Work out the finished part from the listing and answer in its coordinate system (mm). A direction names the side the tool comes from. Coordinates: 2 decimals unless noted, no trailing zeros. Order: outer loops, then holes, each group sorted by start corner. A loop starts at its lowest first (then second) coordinate and runs counter-clockwise, first axis right, second up. Notation, with made-up numbers: M 88,19.25 L 134,19.25 A23 ccw 134,32.25 Z; hole C 82,-23.75 d2. An arc over 180 degrees is marked long. Write item = value, one per line. Start each with the question number.
Q1. Determine the mould class of faces 6 (the cylindrical face through (-8.218, 0.731, 4.825)), 7 (the flat face through (4.02, -0.01, 6.96)), 8 (the flat face through (-4.02, -0.01, 6.96)), 9 (the flat face through (8, 0, 0)) for opening direction X: released by +X, released by -X, zero draft, split by the parting line, or undercut.
Q2. Find section B-B on y = -0.75. Give the vertices of the cut face in (x, z) (3 decimals).
Q3. A tool of negligible diameter and unlimited length cuts with its end or side. For faces 1 (the flat face through (4.02, -0.01, -6.96)), 2 (the cylindrical face through (0, 0, 6.5)), 3 (the flat face through (-0.1, 1, -4.5)), 4 (the flat face through (-8, 0, 0)), 5 (the flat face through (-4.02, -0.01, -6.96)), from which of +Z, -Z, +X, -X, +Y, -Y can it reach the whole face along a straight path? Write none if from no direction.
Q4. Straight lines are drawn through the part: line 1 along Z through (x, y) = (0, 0.3); line 2 along X through (y, z) = (-0.35, -2.5); line 3 along X through (y, z) = (-0.25, -2). For each, find the intervals that lie inside material, in ascending order.
Q5. Find section A-A on x = 0. Give the vertices of the cut face in (y, z), and give its area (3 significant figures).
Q6. Find section D-D on x = 3.5. Give the number of separate pieces and of enclosed holes in the cut face, and give its area (3 significant figures).
Q7. Each of these flat-tipped pins is pushed along its axis until it touches: P1, Ø9, axis at x = 0, z = 0, coming from the -Y side; P2, Ø1, axis at x = -8, y = -0.5, coming from the -Z side. Where does it stop, or does it pass through?
Q8. Find section C-C on z = -3.5. Give the vertices of the cut face in (x, y).
```python
from build123d import *

# Parameters (mm, degrees)
SKETCH005_R          = 9.53
SKETCH005_R_2        = 4
PAD001_DEPTH         = 1
POCKET001_DEPTH      = 55.059013
POCKET001_DEPTH_BACK = 55.059013
POLARPATTERN_COUNT   = 3
SKETCH007_R          = 0.5


with BuildPart() as part:
    # Sketch005 → Pad001 (new body, symmetric)
    with BuildSketch(Plane.XZ):
        Circle(SKETCH005_R)
        Circle(SKETCH005_R_2, mode=Mode.SUBTRACT)
    extrude(amount=PAD001_DEPTH, both=True)

    # Sketch006 → Pocket001 (cut, two sides)
    with BuildSketch(Plane.XZ) as pocket001_sk:
        with BuildLine():
            ThreePointArc((4.765, 8.253222), (0, 9.53), (-4.765, 8.253222))
            Line((-4.765, 8.253222), (-3.25, 5.629165))
            ThreePointArc((3.25, 5.629165), (0, 6.5), (-3.25, 5.629165))
            Line((4.765, 8.253222), (3.25, 5.629165))
        make_face()
    pocket001 = extrude(amount=-POCKET001_DEPTH, mode=Mode.SUBTRACT) + extrude(pocket001_sk.sketch, amount=POCKET001_DEPTH_BACK, mode=Mode.SUBTRACT)

    # PolarPattern: Pocket001 ×3 about axis
    polarpattern_axis = Axis((0, 0, 0), (0, -1, 0))
    for i in range(1, POLARPATTERN_COUNT):
        add(pocket001.rotate(polarpattern_axis, i * 360 / POLARPATTERN_COUNT), mode=Mode.SUBTRACT)

    # Sketch007 → Groove001 (revolve, cut)
    with BuildSketch(Plane.YZ):
        with Locations((0, 9.7)):
            Circle(SKETCH007_R)
    revolve(axis=Axis((0, 0, 0), (0, 1, 0)), mode=Mode.SUBTRACT)


solid = part.part
```
Findings below:
q1.face_6 = released by -X
q1.face_7 = undercut
q1.face_8 = undercut
q1.face_9 = zero draft
q2.outline = M -9.53,0 L -6.5,0 A6.5 ccw -3.25,-5.629 L -4.765,-8.253 A9.53 ccw 4.765,-8.253 L 3.25,-5.629 A6.5 ccw 6.5,0 L 9.53,0 A9.53 ccw 4.765,8.253 L 3.25,5.629 A6.5 ccw -3.25,5.629 L -4.765,8.253 A9.53 ccw Z; hole C 0,0 d8
q3.face_1 = +X, +Y, -Y
q3.face_2 = +Z, +Y, -Y
q3.face_3 = +Z, -Z, +X, -X, +Y
q3.face_4 = -Z, -X, +Y, -Y
q3.face_5 = -X, +Y, -Y
q4.line_1 = -9.3 to -4, 4 to 6.5
q4.line_2 = -6 to -3.12, 3.12 to 6
q4.line_3 = -6.18 to -3.46, 3.46 to 6.18
q5.outline = M -1,-9.53 L -0.47,-9.53 A0.5 cw 0.47,-9.53 L 1,-9.53 L 1,-4 L -1,-4 Z; M -1,4 L 1,4 L 1,6.5 L -1,6.5 Z
q5.area = 15.8 mm^2
q6.separate_pieces = 3
q6.enclosed_holes = 0
q6.area = 20.7 mm^2
q7.P1 = -1
q7.P2 = 0
q8.outline = M -5.48,-1 L -1.94,-1 L -1.94,1 L -5.48,1 Z; M 1.94,-1 L 5.48,-1 L 5.48,1 L 1.94,1 Z
